For this review, take the finished solid that the model builds, in its own axes (mm). Face numbers are marked on the shaded views. A direction names the side the tool comes from. Give positions to 0.01 mm unless a question says otherwise; leave off trailing zeros. Order: outer loops, then holes, each group sorted by start corner. A loop starts at its lowest first (then second) coordinate and runs counter-clockwise, first axis right, second up. Notation, with made-up numbers: (-7.5, 40) - (46.5, 40) arc R18 ccw to (46.5, 57) - close; hole circle Ø1 at (8, 33.25). An arc over 180 degrees is marked (long way). Use a Markdown table: item, result. Add a question column.
1) We need section A-A on z = 11. Write out the cut boundary in (x, y), then the cut area to 3 significant figures.
2) Mouldability with a two-part tool opening along Z and no side actions: class the marked faces 1, 2, 3 and 4 as released by +Z, released by -Z, zero draft, split by the parting line, or undercut.
3) We need section C-C on z = 32. Write out the cut boundary in (x, y), then the cut area to 3 significant figures.
4) Clearance check with flat-ended pins moving along their axes: P1, Ø1.5, axis at y = -45, z = 40.5, coming from the -X side (3 decimals); P2, Ø1, axis at x = 14, z = 7, coming from the +Y side; P3, Ø3, axis at y = -37.5, z = 26.5, coming from the -X side. State where each tip first meets the part, or that it passes through.
5) We need section B-B on y = -69.5. Write out the cut boundary in (x, z).
6) Machinability: for the marked faces 5 and 6, which of the approach directions +Z, -Z, +X, -X, +Y, -Y give a long, thin tool a straight path to every point of the face, cutting with its end or side? Answer none if there is none.
7) We need section D-D on x = 69. Write out the cut boundary in (y, z), then the cut area to 3 significant figures.
8) Wall thickness on L1, parallel to Y at x = 38, z = 31; L2, parallel to X at y = -95, z = 28; L3, parallel to Y at x = 31.5, z = 48: over which ranges is each line inside the solid? List them lowest first.
```python
from build123d import *

# Parameters (mm, degrees)
F0_W     = 76.2
F0_H     = 50.8
F1_DEPTH = 127
F3_DEPTH = 127.001
F4_R     = 12.7
F6_DEPTH = 50.801
F7_SIZE  = 6.35


with BuildPart() as f1:
    # F0 (on Front) → F1 (new body)
    with BuildSketch(Plane.XZ):
        with Locations((38.1, 25.4)):
            Rectangle(F0_W, F0_H)
    extrude(amount=F1_DEPTH)

    # F2 (on face) → F3 (cut, through all)
    with BuildSketch(Plane.XZ.offset(127)):
        with BuildLine():
            ThreePointArc((11.316762, 38.1), (3.239664, 42.294721), (0, 50.8))
            Line((0, 50.8), (0, 0))
            ThreePointArc((0, 0), (3.239664, 8.505279), (11.316762, 12.7))
            ThreePointArc((11.316762, 12.7), (16.214601, 15.24362), (18.179088, 20.401103))
            Line((18.179088, 20.401103), (18.179088, 30.398897))
            ThreePointArc((18.179088, 30.398897), (16.214601, 35.55638), (11.316762, 38.1))
        make_face()
    extrude(amount=-F3_DEPTH, mode=Mode.SUBTRACT)

    # F4
    f4_edges = [f1.edges().sort_by_distance(p)[0] for p in [
        (76.2, -63.5, 50.8),
        (76.2, -63.5, 0),
    ]]
    fillet(f4_edges, radius=F4_R)

    # F5 (on face) → F6 (cut, through all)
    with BuildSketch(Plane(origin=(0, 0, 0), x_dir=(1, 0, 0), z_dir=(0, 0, -1))):
        with BuildLine():
            ThreePointArc((38.1, 88.9), (42.590128, 90.759872), (44.45, 95.25))
            ThreePointArc((44.45, 95.25), (33.609872, 99.740128), (38.1, 88.9))
        make_face()
        with BuildLine():
            ThreePointArc((44.45, 31.75), (42.590128, 36.240128), (38.1, 38.1))
            ThreePointArc((38.1, 38.1), (33.609872, 27.259872), (44.45, 31.75))
        make_face()
    extrude(amount=-F6_DEPTH, mode=Mode.SUBTRACT)

    # F7
    f7_edges = [f1.edges().sort_by_distance(p)[0] for p in [
        (38.1, -101.6, 50.8),
        (31.75, -31.75, 50.8),
    ]]
    chamfer(f7_edges, length=F7_SIZE)


solid = f1.part
```
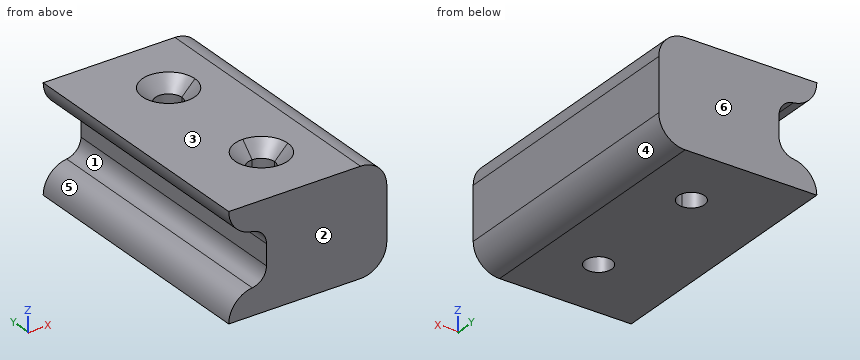
Checked values:
| question | item | result |
|---|---|---|
| 1 | outline | (6.27, -127) - (76.09, -127) - (76.09, 0) - (6.27, 0) - close; hole circle Ø12.7 at (38.1, -95.25); hole circle Ø12.7 at (38.1, -31.75) |
| 1 | area | 8,610 mm² |
| 2 | face 1 | undercut |
| 2 | face 2 | zero draft |
| 2 | face 3 | released by +Z |
| 2 | face 4 | released by -Z |
| 3 | outline | (18.01, -127) - (76.2, -127) - (76.2, 0) - (18.01, 0) - close; hole circle Ø12.7 at (38.1, -95.25); hole circle Ø12.7 at (38.1, -31.75) |
| 3 | area | 7,140 mm² |
| 4 | P1 | x = 4.285 |
| 4 | P2 | y = 0 |
| 4 | P3 | x = 18.18 |
| 5 | outline | (0, 0) - (63.5, 0) arc R12.7 ccw to (76.2, 12.7) - (76.2, 38.1) arc R12.7 ccw to (63.5, 50.8) - (0, 50.8) arc R12.78 ccw to (11.32, 38.1) arc R7.75 cw to (18.18, 30.4) - (18.18, 20.4) arc R7.75 cw to (11.32, 12.7) arc R12.78 ccw to start |
| 6 | face 5 | -X, +Y, -Y |
| 6 | face 6 | +Z, -Z, +X, -X, +Y |
| 7 | outline | (-127, 1.25) - (0, 1.25) - (0, 49.55) - (-127, 49.55) - close |
| 7 | area | 6,130 mm² |
| 8 | L1 | -127 to -101.6, -88.9 to -38.1, -25.4 to 0 |
| 8 | L2 | 18.18 to 31.75, 44.45 to 76.2 |
| 8 | L3 | -127 to -102.63, -87.87 to -39.13, -24.37 to 0 |
